The model under review builds one solid part; all positions refer to its coordinate system, in mm. Round coordinates to 2 decimals unless told otherwise and drop trailing zeros. Write each loop counter-clockwise with the first axis right and the second up, starting at its lowest first coordinate (ties: lowest second). Pieces come first, ordered by that corner, then holes. Notation, with made-up numbers: (21, 32.5) -> (52, 32.5) arc R13 ccw to (52, 50.5) -> close; hole circle Ø3 at (-17, -26.5). An arc over 180 degrees is marked (long way). Use CSV: the item, a comma, the result in double quotes. Start each with the question number.
1) For pin 1 Ø0.7 at (x, z) = (1, 0) entering from +Y; pin 2 Ø0.7 at (x, z) = (0.5, 4) entering from -Y, all flat-tipped, find the tip position at first contact; note any pin that passes through.
2) Take a section at B-B, the plane z = -6. Give the boundary of the cut face in (x, y).
3) Take a section at C-C, the plane x = 1.1. State how many separate pieces and enclosed holes the cut face has, then the cut area to 3 significant figures.
4) Wall thickness on probe 1 along Z at (x, y) = (0.15, 6.5); probe 2 along Z at (x, y) = (0.7, 6); probe 3 along Y at (x, z) = (0.45, -5): over which ranges is each line inside the solid? List them lowest first. Write a range as [from, to].
5) Take a section at A-A, the plane z = 0. Give the boundary of the cut face in (x, y).
from build123d import *

# Parameters (mm, degrees)
SCHIZZO1_R                   = 1.5
ESTRUSIONE_ESTRUSIONE1_DEPTH = 1.35
RACCORDO2_R                  = 3
RACCORDO3_R                  = 3
RACCORDO4_R                  = 0.7


with BuildPart() as part:
    # Schizzo1 → Estrusione-Estrusione1 (new body)
    with BuildSketch(Plane(origin=(0, 0, 0), x_dir=(0, 0, -1), z_dir=(1, 0, 0))):
        with BuildLine():
            add(Edge.make_bspline(
                [(-7.501010101, -10.3), (-10.845030199, -9.13986581), (-13.865102381, -7.304364218), (-17.601010101, -6.594005849)],
                knots=[0.271280726, 0.271280726, 0.271280726, 0.271280726, 0.852483684, 0.852483684, 0.852483684, 0.852483684], degree=3))
            add(Edge.make_bspline(
                [(-2.501010101, -11.3), (-4.308742426, -11.235865063), (-5.940164296, -10.841501107), (-7.501010101, -10.3)],
                knots=[0, 0, 0, 0, 0.271280726, 0.271280726, 0.271280726, 0.271280726], degree=3))
            Line((-2.501010101, -11.3), (1.498989899, -11.3))
            ThreePointArc((1.498989899, -11.3), (11.398989899, 0), (1.498989899, 11.3))
            Line((1.498989899, 11.3), (-2.501010101, 11.3))
            add(Edge.make_bspline(
                [(-2.501010101, 11.3), (-4.209338931, 11.338090952), (-5.850739142, 10.914740779), (-7.501010101, 10.3)],
                knots=[0, 0, 0, 0, 0.293888871, 0.293888871, 0.293888871, 0.293888871], degree=3))
            add(Edge.make_bspline(
                [(-7.501010101, 10.3), (-10.658273676, 9.123890914), (-13.848006436, 7.247243694), (-17.601010101, 6.561146452)],
                knots=[0.293888871, 0.293888871, 0.293888871, 0.293888871, 0.856150858, 0.856150858, 0.856150858, 0.856150858], degree=3))
            Line((-17.601010101, 6.561146452), (-17.601010101, 0))
            Line((-17.601010101, 0), (-17.601010101, -6.594005849))
        make_face()
        with Locations(Location((5, -6, 0), (0, 0, 180))):
            Circle(SCHIZZO1_R, mode=Mode.SUBTRACT)
        with BuildLine():
            ThreePointArc((-10.5, 0), (-12, -1.5), (-13.5, 0))
            ThreePointArc((-13.5, 0), (-12, 1.5), (-10.5, 0))
        make_face(mode=Mode.SUBTRACT)
        Polygon((-7.9, -3.5), (-7.9, 0), (-7.9, 3.5), (-1.901010101, 3.5), (-1.901010101, 8.4), (1.898989899, 8.4), (1.898989899, 3.5), (7.898989899, 3.5), (7.898989899, -3.5), (1.898989899, -3.5), (1.898989899, -8.4), (-1.901010101, -8.4), (-1.901010101, -3.5), align=None, mode=Mode.SUBTRACT)
        with Locations(Location((5, 6, 0), (0, 0, 180))):
            Circle(SCHIZZO1_R, mode=Mode.SUBTRACT)
    extrude(amount=ESTRUSIONE_ESTRUSIONE1_DEPTH)

    # Raccordo2
    raccordo2_edges = [part.edges().sort_by_distance(p)[0] for p in [
        (0.675, -6.594005849, 17.601010101),
    ]]
    fillet(raccordo2_edges, radius=RACCORDO2_R)

    # Raccordo3
    raccordo3_edges = [part.edges().sort_by_distance(p)[0] for p in [
        (0.675, 6.561146452, 17.601010101),
    ]]
    fillet(raccordo3_edges, radius=RACCORDO3_R)

    # Raccordo4
    raccordo4_edges = [part.edges().sort_by_distance(p)[0] for p in [
        (0.675, -3.5, 1.901010101),
        (0.675, -8.4, 1.901010101),
        (0.675, -8.4, -1.898989899),
        (0.675, -3.5, -1.898989899),
        (0.675, -3.5, -7.898989899),
        (0.675, 3.5, -7.898989899),
        (0.675, 3.5, -1.898989899),
        (0.675, 8.4, -1.898989899),
        (0.675, 8.4, 1.901010101),
        (0.675, 3.5, 1.901010101),
        (0.675, 3.5, 7.9),
        (0.675, -3.5, 7.9),
    ]]
    fillet(raccordo4_edges, radius=RACCORDO4_R)


solid = part.part
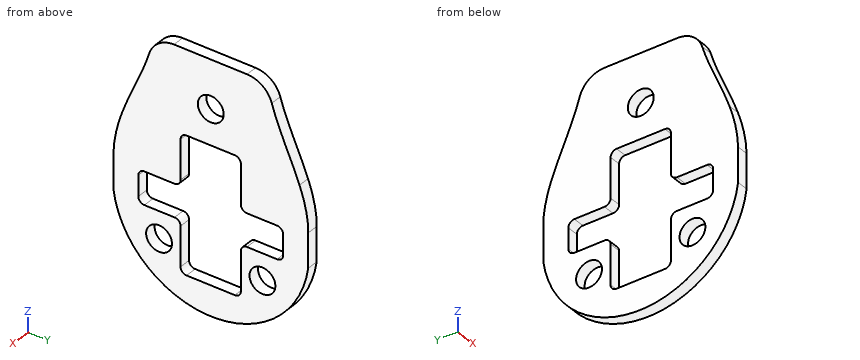
Values found:
1,pin 1,"y = 11.3"
1,pin 2,"y = -11.21"
2,outline,"(0, -9.69) -> (1.35, -9.69) -> (1.35, -7.12) -> (0, -7.12) -> close; (0, -4.88) -> (1.35, -4.88) -> (1.35, -3.5) -> (0, -3.5) -> close; (0, 3.5) -> (1.35, 3.5) -> (1.35, 4.88) -> (0, 4.88) -> close; (0, 7.12) -> (1.35, 7.12) -> (1.35, 9.69) -> (0, 9.69) -> close"
3,separate pieces,"1"
3,enclosed holes,"4"
3,area,"366 mm²"
4,probe 1,"[-9.36, -6.41], [-3.59, -1.9], [1.9, 16.54]"
4,probe 2,"[-9.69, -6.5], [-3.5, -1.9], [1.9, 17.01]"
4,probe 3,"[-10.24, -7.5], [-4.5, -3.5], [3.5, 4.5], [7.5, 10.24]"
5,outline,"(0, -11.3) -> (1.35, -11.3) -> (1.35, -8.4) -> (0, -8.4) -> close; (0, 8.4) -> (1.35, 8.4) -> (1.35, 11.3) -> (0, 11.3) -> close"
